from build123d import *

# Parameters (mm, degrees)
SKETCH1_R           = 20
BOSS_EXTRUDE1_DEPTH = 1
SKETCH2_W           = 13.037346626
SKETCH2_H           = 1.230994102
CUT_EXTRUDE1_DEPTH  = 1
SKETCH3_R           = 1
CUT_EXTRUDE2_DEPTH  = 1


with BuildPart() as part:
    # Sketch1 → Boss-Extrude1 (new body)
    with BuildSketch(Plane.XY):
        Circle(SKETCH1_R)
    extrude(amount=BOSS_EXTRUDE1_DEPTH)

    # Sketch2 → Cut-Extrude1 (cut)
    with BuildSketch(Plane.XY.offset(1)):
        with Locations((0, -14.296317866)):
            Rectangle(SKETCH2_W, SKETCH2_H)
        with Locations((0, 14.296317866)):
            Rectangle(SKETCH2_W, SKETCH2_H)
    extrude(amount=-CUT_EXTRUDE1_DEPTH, mode=Mode.SUBTRACT)

    # Sketch3 → Cut-Extrude2 (cut)
    with BuildSketch(Plane.XY.offset(1)):
        Circle(SKETCH3_R)
    extrude(amount=-CUT_EXTRUDE2_DEPTH, mode=Mode.SUBTRACT)


solid = part.part
Work out the finished part from the listing and answer in its coordinate system (mm). A direction names the side the tool comes from. Give positions to 0.01 mm unless a question says otherwise; leave off trailing zeros. Write each loop counter-clockwise with the first axis right and the second up, starting at its lowest first coordinate (ties: lowest second). Pieces come first, ordered by that corner, then holes. Notation, with made-up numbers: M -18,23.5 L -5,23.5 A25 cw -5,62.5 Z; hole C 65.25,80 d6. An arc over 180 degrees is marked long. Answer as CSV lines item,"result".
Q1. A cutting plane is placed at D-D on x = 5. Write down the section's boundary in (y, z), plus the area to 3 significant figures.
A:
outline,"M -19.36,0 L -14.91,0 L -14.91,1 L -19.36,1 Z; M -13.68,0 L 13.68,0 L 13.68,1 L -13.68,1 Z; M 14.91,0 L 19.36,0 L 19.36,1 L 14.91,1 Z"
area,"36.3 mm²"
Q2. The mould has two halves that part along X. Classify faces 3 (the flat face through (-0.1, 14.912, 0.5)), 4 (the flat face through (4, 0, 1)), 5 (the cylindrical face through (-4.336, -19.524, 0.493)), 6 (the flat face through (6.519, 14.3, 0.5)): +X half, -X half, draft (parallel to the pull), parting line (faces both ways), or undercut.
A:
face 3,"undercut"
face 4,"draft"
face 5,"parting line"
face 6,"undercut"
Q3. Given P1, Ø0.5, axis at x = -2.5, z = 0.5, coming from the -Y side, flat-ended and moving along its own axis, determine where the tip first touches the part or whether it passes through.
A:
P1,"stops at y = -19.87"
Q4. A cutting plane is placed at A-A on x = 0. Write down the section's boundary in (y, z).
A:
outline,"M -20,0 L -14.91,0 L -14.91,1 L -20,1 Z; M -13.68,0 L -1,0 L -1,1 L -13.68,1 Z; M 1,0 L 13.68,0 L 13.68,1 L 1,1 Z; M 14.91,0 L 20,0 L 20,1 L 14.91,1 Z"
Q5. A cutting plane is placed at C-C on z = 0.6. Write down the section's boundary in (x, y), plus the area to 3 significant figures.
A:
outline,"C 0,0 d40; hole M -6.52,-14.91 L 6.52,-14.91 L 6.52,-13.68 L -6.52,-13.68 Z; hole M -6.52,13.68 L 6.52,13.68 L 6.52,14.91 L -6.52,14.91 Z; hole C 0,0 d2"
area,"1,220 mm²"
Q6. A cutting plane is placed at B-B on y = 0. Write down the section's boundary in (x, z).
A:
outline,"M -20,0 L -1,0 L -1,1 L -20,1 Z; M 1,0 L 20,0 L 20,1 L 1,1 Z"
Q7. Find the intervals of material crossed by probe 1 along Y at (x, z) = (0, 0.7); probe 2 along Y at (x, z) = (-3, 0.85); probe 3 along Y at (x, z) = (6, 0.4), in increasing order. Write a range as [from, to].
A:
probe 1,"y = [-20, -14.91], [-13.68, -1], [1, 13.68], [14.91, 20]"
probe 2,"y = [-19.77, -14.91], [-13.68, 13.68], [14.91, 19.77]"
probe 3,"y = [-19.08, -14.91], [-13.68, 13.68], [14.91, 19.08]"
Q8. A tool of negligible diameter and unlimited length cuts with its end or side. For faces 1 (the flat face through (-0.1, -14.912, 0.5)), 2 (the flat face through (4, 0, 0)), from which of +Z, -Z, +X, -X, +Y, -Y can it reach the whole face along a straight path? Write none if from no direction.
A:
face 1,"+Z, -Z"
face 2,"-Z, +X, -X, +Y, -Y"
